Verification items for the finished model (mm, model axes). A direction names the side the tool comes from. Coordinates: 2 decimals unless noted, no trailing zeros. Order: outer loops, then holes, each group sorted by start corner. A loop starts at its lowest first (then second) coordinate and runs counter-clockwise, first axis right, second up. Notation, with made-up numbers: (-33, 20) -> (17, 20) arc R32 ccw to (17, 58) -> close; hole circle Ø10 at (38.5, 72.5). An arc over 180 degrees is marked (long way). Use CSV: the item, a comma, the result in double quotes. Start each with the question number.
1) Sectioned sample at B-B on x = 0. Record the boundary of the cut face in (y, z), then the cut area to 3 significant figures.
2) Sectioned sample at A-A on y = -5.25. Record the boundary of the cut face in (x, z).
3) Sectioned sample at C-C on y = 0.5. Record the boundary of the cut face in (x, z), then the cut area to 3 significant figures.
4) Sectioned sample at D-D on z = 5. Record the boundary of the cut face in (x, y), then the cut area to 3 significant figures.
5) Tool access check on faces 5 (the flat face through (-3.176, 3.299, 1.507)), 6 (the flat face through (-2, -4.5, 12)), 7 (the flat face through (2, -5.5, 6)). Record the directions out of +Z, -Z, +X, -X, +Y, -Y that give a thin tool (end or side, any length) a straight path to the whole face; none if there is none.
6) Go/stop test with flat-tipped pins: pin 1 (1 mm diameter, centred on x = 0, z = 4.5, fed in from +Y); pin 2 (2.5 mm diameter, centred on x = 1.5, z = 9.5, fed in from +Y); pin 3 (2 mm diameter, centred on x = -2.5, y = 3.5, fed in from +Z). Record where each tip stops, or that it passes through.
7) Scan lines: line 1 along X through (y, z) = (-6.25, 8); line 2 along Y through (x, z) = (0, 0.8); line 3 along Z through (x, y) = (0, -6.15). Record each from-to range of solid material in increasing order.
8) Release check for a two-part mould opening along Y. For faces 1 (the flat face through (0, 6.5, 1)), 2 (the flat face through (3.176, -0.299, 1.507)), 3 (the flat face through (0, 5.15, 1.5)), 4 (the flat face through (0, -1, 0)) record: released by +Y, released by -Y, zero draft, split by the parting line, or undercut.
Autodesk Inventor part; units mm, degrees
ref_plane "YZ Plane" through (0, 0, 0) normal (1, 0, 0) x (0, 1, 0)
ref_plane "XZ Plane" through (0, 0, 0) normal (0, 1, 0) x (-1, 0, 0)
ref_plane "XY Plane" through (0, 0, 0) normal (0, 0, 1) x (1, 0, 0)
sketch "Sketch1" plane through (0, 0, 0) normal (0, 0, 1) x (1, 0, 0)
  line L0 (-5, -6.5) -> (5, -6.5)
  line L1 (5, -6.5) -> (5, 6.5)
  line L2 (5, 6.5) -> (-5, 6.5)
  line L3 (-5, 6.5) -> (-5, -6.5)
  line L4 (-5, -6.5) -> (5, 6.5) construction
  line L5 (5, -6.5) -> (-5, 6.5) construction
  circle A0 centre (0, 1.5) radius 2.1
  point P0 (0, 0)
  dimension "d0" = 10
  dimension "d1" = 13
  dimension "d2" = 4.2
  dimension "d3" = 5
  dimension "d4" = 5
extrude "Extrusion1" add sketch "Sketch1" along normal blind 2
sketch "Sketch2" plane through (-5, -6.5, 0) normal (0, -1, 0) x (1, 0, 0)
  line L0 (0, 0) -> (10, 0)
  line L1 (10, 0) -> (10, 13)
  line L2 (10, 13) -> (0, 13)
  line L3 (0, 13) -> (0, 0)
  circle A0 centre (5, 8) radius 2.1
  point P0 (5, 0)
  dimension "d7" = 10
  dimension "d8" = 13
  dimension "d9" = 5
  dimension "d10" = 13
  dimension "d11" = 4.2
  dimension "d12" = 5
  dimension "d13" = 5
extrude "Extrusion2" add sketch "Sketch2" against normal blind 2
sketch "Sketch3" plane through (-5, -4.5, 0) normal (0, 1, 0) x (1, 0, 0)
  circle A0 centre (5, -8) radius 2.1
  line L0 (9.2147, -8) -> (7.1073, -11.65)
  line L1 (7.1073, -11.65) -> (2.8927, -11.65)
  line L2 (2.8927, -11.65) -> (0.7853, -8)
  line L3 (0.7853, -8) -> (2.8927, -4.35)
  line L4 (2.8927, -4.35) -> (7.1073, -4.35)
  line L5 (7.1073, -4.35) -> (9.2147, -8)
  point P0 (5, 0)
  dimension "d16" = 7.3
extrude "Extrusion3" cut sketch "Sketch3" against normal blind 1
sketch "Sketch4" plane through (0, 0, 2) normal (0, 0, 1) x (1, 0, 0)
  circle A0 centre (0, 1.5) radius 2.1
  line L0 (4.2147, 1.5) -> (2.1073, -2.15)
  line L1 (2.1073, -2.15) -> (-2.1073, -2.15)
  line L2 (-2.1073, -2.15) -> (-4.2147, 1.5)
  line L3 (-4.2147, 1.5) -> (-2.1073, 5.15)
  line L4 (-2.1073, 5.15) -> (2.1073, 5.15)
  line L5 (2.1073, 5.15) -> (4.2147, 1.5)
  point P0 (0, 0)
  dimension "d19" = 7.3
extrude "Extrusion4" cut sketch "Sketch4" against normal blind 1
fillet "Fillet1" radius 2 4 edges at (-5, 6.5, 1) (5, 6.5, 1) (5, -5.5, 13) (-5, -5.5, 13)
fillet "Fillet2" radius 2 1 edges at (0, -4.5, 2)
properties part number "24 bevestigings hoekjes 2 kanten"
Answers follow:
1,outline,"(-6.5, 0) -> (-0.6, 0) -> (-0.6, 1) -> (-2.15, 1) -> (-2.15, 2) -> (-2.5, 2) arc R2 cw to (-4.5, 4) -> (-4.5, 4.35) -> (-5.5, 4.35) -> (-5.5, 5.9) -> (-6.5, 5.9) -> close; (-6.5, 10.1) -> (-5.5, 10.1) -> (-5.5, 11.65) -> (-4.5, 11.65) -> (-4.5, 13) -> (-6.5, 13) -> close; (3.6, 0) -> (6.5, 0) -> (6.5, 2) -> (5.15, 2) -> (5.15, 1) -> (3.6, 1) -> close"
1,area,"25.9 mm²"
2,outline,"(-5, 0) -> (5, 0) -> (5, 11) arc R2 ccw to (3, 13) -> (-3, 13) arc R2 ccw to (-5, 11) -> close; hole (-4.21, 8) -> (-2.11, 4.35) -> (2.11, 4.35) -> (4.21, 8) -> (2.11, 11.65) -> (-2.11, 11.65) -> close"
3,outline,"(-5, 0) -> (-1.85, 0) -> (-1.85, 1) -> (-3.64, 1) -> (-3.64, 2) -> (-5, 2) -> close; (1.85, 0) -> (5, 0) -> (5, 2) -> (3.64, 2) -> (3.64, 1) -> (1.85, 1) -> close"
3,area,"9.03 mm²"
4,outline,"(-5, -6.5) -> (5, -6.5) -> (5, -4.5) -> (2.48, -4.5) -> (2.48, -5.5) -> (-2.48, -5.5) -> (-2.48, -4.5) -> (-5, -4.5) -> close"
4,area,"15.0 mm²"
5,face 5,"+Z"
5,face 6,"+Z, +X, -X, +Y"
5,face 7,"+Y"
6,pin 1,"stops at y = -4.5"
6,pin 2,"stops at y = -5.5"
6,pin 3,"stops at z = 2"
7,line 1,"x = -5 to -2.1, 2.1 to 5"
7,line 2,"y = -6.5 to -0.6, 3.6 to 6.5"
7,line 3,"z = 0 to 5.9, 10.1 to 13"
8,face 1,"released by +Y"
8,face 2,"undercut"
8,face 3,"undercut"
8,face 4,"zero draft"
